Source: CAD feature listing. Evaluate the final solid. Frame: model axes, mm. Face numbers are marked on the shaded views. A direction names the side the tool comes from. Give positions to 0.01 mm unless a question says otherwise; leave off trailing zeros. Loops run counter-clockwise (first coordinate to the right, second up) from the corner with the lowest first, then second, coordinate; pieces in that order, holes last. Notation, with made-up numbers: (83, -3.5) -> (122, -3.5) arc R20 ccw to (122, 9.5) -> close; hole circle Ø7 at (73, 40.25). An arc over 180 degrees is marked (long way). Put each result on its own line as item: value.
```python
from build123d import *


with BuildPart() as f1:
    # F0 (on Top) → F1 (revolve)
    with BuildSketch(Plane.XY):
        with BuildLine():
            ThreePointArc((-105.669873, 95.5), (-107.5, 97.330127), (-110, 98))
            Line((-110, 98), (-195, 98))
            Line((-195, 98), (-195, 113))
            Line((-195, 113), (-200, 113))
            Line((-200, 113), (-200, 98))
            Line((-200, 98), (-200, 78))
            Line((-200, 78), (-152, 78))
            Line((-152, 78), (-152, 89))
            Line((-152, 89), (0, 89))
            Line((0, 89), (0, 93))
            Line((0, 93), (-101.339746, 93))
            ThreePointArc((-101.339746, 93), (-103.839746, 93.669873), (-105.669873, 95.5))
        make_face()
        with BuildLine():
            Line((101.339746, 93), (0, 93))
            Line((0, 93), (0, 89))
            Line((0, 89), (152, 89))
            Line((152, 89), (152, 78))
            Line((152, 78), (200, 78))
            Line((200, 78), (200, 98))
            Line((200, 98), (200, 113))
            Line((200, 113), (195, 113))
            Line((195, 113), (195, 98))
            Line((195, 98), (110, 98))
            ThreePointArc((110, 98), (107.5, 97.330127), (105.669873, 95.5))
            ThreePointArc((105.669873, 95.5), (103.839746, 93.669873), (101.339746, 93))
        make_face()
    revolve(axis=Axis((-6.106503, 0, 0), (1, 0, 0)))


solid = f1.part
```
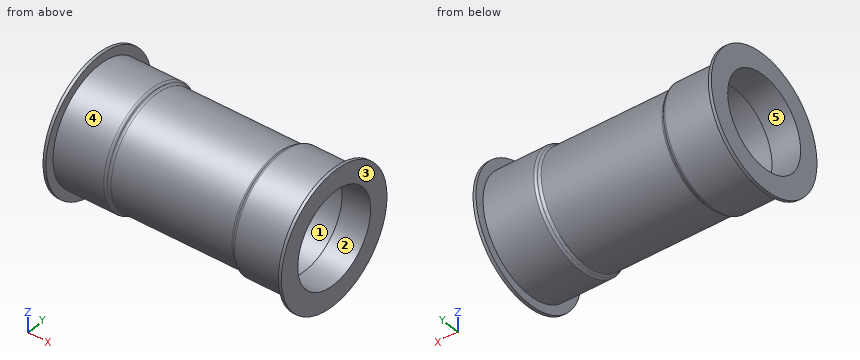
(1) Reachability of the marked faces 1 and 2 from +Z, -Z, +X, -X, +Y, -Y: full face, straight path, thin tool, end or side. Return the list, or none.
Calculated:
face 1: none
face 2: +X, -X
(2) First-contact query: P1, Ø2, axis at x = -158, z = -79, coming from the -Y side; P2, Ø3, axis at x = -1.5, z = 7, coming from the -Y side; P3, Ø4, axis at x = -47, z = 12.5, coming from the -Y side. Flat tips, straight axial feed; report the tip coordinate or a pass-through.
Calculated:
P1: stops at y = -59.33
P2: stops at y = -92.84
P3: stops at y = -92.41
(3) Section A-A on x = 1.5. Return loops of the section in (y, z), then the cut area to 3 significant figures.
Calculated:
outline: circle Ø186 at (0, 0); hole circle Ø178 at (0, 0)
area: 2,290 mm²
(4) Draft query along Z for the marked faces 3, 4 and 5. Return one class per face: released by +Z, released by -Z, zero draft, split by the parting line, or undercut.
Calculated:
face 3: zero draft
face 4: split by the parting line
face 5: undercut
(5) Line query: probe 1 along X at (y, z) = (-57, -80.5); probe 2 along Z at (x, y) = (179, 0); probe 3 along Y at (x, z) = (-115, -20.5). Output: solid intervals per line, ascending. Write a range as from..to.
Calculated:
probe 1: x = -200..-195, 195..200
probe 2: z = -98..-78, 78..98
probe 3: y = -95.83..-86.61, 86.61..95.83
(6) Section B-B on x = 147. Return loops of the section in (y, z), then the cut area to 3 significant figures.
Calculated:
outline: circle Ø196 at (0, 0); hole circle Ø178 at (0, 0)
area: 5,290 mm²
